```python
from build123d import *

# Parameters (mm, degrees)
SKETCH1_R           = 35.5
BOSS_EXTRUDE1_DEPTH = 15
CUT_EXTRUDE2_REACH  = 54.398
BOSS_EXTRUDE2_REACH = 64.398
BOSS_EXTRUDE2_START = -10
CUT_EXTRUDE3_START  = -36
SKETCH5_W           = 10.5
SKETCH5_H           = 5.5
CUT_EXTRUDE3_DEPTH  = 22
CHAMFER1_SIZE       = 0.6
CHAMFER2_SIZE       = 2
CUT_EXTRUDE4_REACH  = 58.085
SKETCH6_R           = 3


with BuildPart() as part:
    # Sketch1 → Boss-Extrude1 (new body)
    with BuildSketch(Plane.XY):
        Circle(SKETCH1_R)
    extrude(amount=BOSS_EXTRUDE1_DEPTH)

    # Sketch2 → Cut-Revolve3 (revolve, cut)
    with BuildSketch(Plane(origin=(0, 0, 0), x_dir=(1, 0, 0), z_dir=(0, 1, 0)), mode=Mode.PRIVATE) as cut_revolve3_sk:
        Polygon((-35.5, 0), (-0.1, 0), (-35.5, -10), align=None)
        Polygon((-0.1, -15), (-0.1, -5), (-35.5, -15), align=None)
    revolve(cut_revolve3_sk.sketch.rotate(Axis((0, 0, 0), (0, 0, 1)), 180), axis=Axis((0, 0, 0), (0, 0, 1)), mode=Mode.SUBTRACT)

    # Sketch3 → Cut-Extrude2 (cut, up to next)
    with BuildSketch(Plane.XY, mode=Mode.PRIVATE) as cut_extrude2_sk1:
        with BuildLine():
            Line((6, 35.5), (6, 0))
            ThreePointArc((6, 0), (0, -6), (-6, 0))
            Line((-6, 0), (-6, 35.5))
            ThreePointArc((-6, 35.5), (0, 41.5), (6, 35.5))
        make_face()
    cut_extrude2_tool1 = extrude(cut_extrude2_sk1.sketch, amount=CUT_EXTRUDE2_REACH, mode=Mode.PRIVATE) & part.part
    add(cut_extrude2_tool1.solids().sort_by_distance((0, 17.75, 0))[0], mode=Mode.SUBTRACT)

    # Boss-Extrude2: up to this cone (the profile starts outside it)
    boss_extrude2_end = Plane(origin=(0, 0, -10), z_dir=(0, 0, 1)).offset(9.971752412) * Cone(3.54e-06, 194.43892, 54.926247588, align=(Align.CENTER, Align.CENTER, Align.MIN), mode=Mode.PRIVATE)
    # Sketch4 → Boss-Extrude2 (add, up to the surface)
    with BuildSketch(Plane.XY.offset(BOSS_EXTRUDE2_START), mode=Mode.PRIVATE) as boss_extrude2_sk1:
        with BuildLine():
            Line((-8.175, -9.370902434), (8.175, -9.370902434))
            Line((8.175, -9.370902434), (8.175, -34.545902434))
            ThreePointArc((8.175, -34.545902434), (0, -35.5), (-8.175, -34.545902434))
            Line((-8.175, -34.545902434), (-8.175, -9.370902434))
        make_face()
    boss_extrude2_tool1 = extrude(boss_extrude2_sk1.sketch, amount=BOSS_EXTRUDE2_REACH, mode=Mode.PRIVATE) - boss_extrude2_end
    add(boss_extrude2_tool1.solids().sort_by_distance((0, -22.278861, -10))[0])

    # Sketch5 → Cut-Extrude3 (cut)
    with BuildSketch(Plane(origin=(0, 0, 0), x_dir=(1, 0, 0), z_dir=(0, 1, 0)).offset(CUT_EXTRUDE3_START)):
        with Locations((0, 2.75)):
            Rectangle(SKETCH5_W, SKETCH5_H)
    extrude(amount=CUT_EXTRUDE3_DEPTH, mode=Mode.SUBTRACT)

    # Chamfer1
    chamfer1_edges = [part.edges().sort_by_distance(p)[0] for p in [
        (-5.25, -24.554824835, -5.5),
        (-5.25, -24.554824835, 0),
        (5.25, -24.554824835, 0),
        (5.25, -24.554824835, -5.5),
    ]]
    chamfer(chamfer1_edges, length=CHAMFER1_SIZE)

    # Chamfer2
    chamfer2_edges = [part.edges().sort_by_distance(p)[0] for p in [
        (8.175, -9.370902434, -3.257681969),
        (-8.175, -9.370902434, -3.257681969),
        (8.175, -21.958402434, -10),
        (0, -9.370902434, -10),
        (-8.175, -21.958402434, -10),
    ]]
    chamfer(chamfer2_edges, length=CHAMFER2_SIZE)

    # Sketch6 → Cut-Extrude4 (cut, up to next)
    with BuildSketch(Plane(origin=(0, 0, -10), x_dir=(-1, 0, 0), z_dir=(0, 0, -1)), mode=Mode.PRIVATE) as cut_extrude4_sk1:
        with Locations((0, -21)):
            Circle(SKETCH6_R)
    cut_extrude4_tool1 = extrude(cut_extrude4_sk1.sketch, amount=-CUT_EXTRUDE4_REACH, mode=Mode.PRIVATE) & part.part
    add(cut_extrude4_tool1.solids().sort_by_distance((0, -21, -10))[0], mode=Mode.SUBTRACT)


solid = part.part
```
Can you work these out from the model? Positions are in its coordinate system, mm. A direction names the side the tool comes from. Coordinates: 2 decimals unless noted, no trailing zeros. Loops run counter-clockwise (first coordinate to the right, second up) from the corner with the lowest first, then second, coordinate; pieces in that order, holes last. Notation, with made-up numbers: (-33, 29.5) -> (-20, 29.5) arc R35 cw to (-20, 66.5) -> close; hole circle Ø4 at (39.25, -0.5). An arc over 180 degrees is marked (long way). Answer as a JSON object with one key per item and string values.
1) For faces 1 (the face through (-5.25, -25, -3)), 2 (the face through (-8.175, -23, -1)), 3 (the face through (-6, 17, 8)), 4 (the face through (-7.161, -10.357, -2.12)), which set-ups out of +Z, -Z, +X, -X, +Y, -Y let a thin tool reach every point of the face, with its end or its side?
Results:
{"face 1": "-Y", "face 2": "-Z, -X, -Y", "face 3": "+Z, -Z, +Y", "face 4": "-Z, -X"}
2) Imagine slicing it at A-A (x = 0). Please give me the cut outline in (y, z).
Results:
{"outline": "(-35.5, -10) -> (-24, -10) -> (-24, -5.5) -> (-35.5, -5.5) -> close; (-35.5, 0) -> (-14, 0) -> (-14, -5.5) -> (-18, -5.5) -> (-18, -10) -> (-11.37, -10) -> (-9.37, -8) -> (-9.37, 2.62) -> (-6, 1.67) -> (-6, 6.67) -> (-35.5, 15) -> close"}
3) If I drill on line 1 (Y direction, x = 0, z = -6.9); line 2 (Y direction, x = 0, z = -8.4); line 3 (X direction, y = 30.5, z = 11.5), over which ranges is the centre line in solid material (lowest first)?
Results:
{"line 1": "y = -35.5 to -24, -18 to -9.37", "line 2": "y = -35.5 to -24, -18 to -9.77", "line 3": "x = -18.17 to -6, 6 to 18.17"}
4) For P1, Ø10.5, axis at y = 23, z = 5, coming from the -X side; P2, Ø10.5, axis at y = 12, z = 5, coming from the +X side; P3, Ø1, axis at x = -22.5, y = 12.5, coming from the +Z side, each with a flat end and sliding along its axis, tell me the tip position at first contact or that it passes through.
Results:
{"P1": "stops at x = -28.33", "P2": "stops at x = 33.94", "P3": "stops at z = 12.38"}
5) Thinking about a two-plate mould opening in Z: for faces 5 (the face through (6, 18, 8)), 6 (the face through (0, -25, -5.5)), 7 (the face through (7.32, 2.83, 2.19)), which applies, pulls with the +Z half, pulls with the -Z half, needs draft (parallel to the pull), parting line crosses it, or undercut?
Results:
{"face 5": "needs draft", "face 6": "undercut", "face 7": "pulls with the -Z half"}
